from build123d import *

# Parameters (mm, degrees)
ESBO_O1_R                = 1.6
ESBO_O1_R_2              = 5.15
ESBO_O1_W                = 14.5
ESBO_O1_H                = 10
ESBO_O1_W_2              = 30.747802568
ESBO_O1_H_2              = 3
ESBO_O1_W_3              = 30.747802569
RESSALTO_EXTRUS_O1_DEPTH = 7
RESSALTO_EXTRUS_O3_START = 7
ESBO_O1_5_W              = 30.747802569
ESBO_O1_5_H              = 3
ESBO_O1_5_W_2            = 30.747802568
RESSALTO_EXTRUS_O3_DEPTH = 5


with BuildPart() as part:
    # Esboço1 → Ressalto-extrusão1 (new body)
    # profile 1 of 5: a face of its own
    with BuildSketch(Plane.XY):
        Polygon((60.087398189, 33.548797322), (-59.912601811, 33.548797322), (-59.912601811, 26.644004496), (-29.164799242, 26.644004496), (-29.164799242, 23.644004496), (-59.912601811, 23.644004496), (-59.912601811, -30.686339735), (-29.164799242, -30.686339735), (-29.164799242, -33.686339735), (-59.912601811, -33.686339735), (-59.912601811, -40.591132561), (60.087398189, -40.591132561), (60.087398189, -33.686339735), (29.339595621, -33.686339735), (29.339595621, -30.686339735), (60.087398189, -30.686339735), (60.087398189, 23.644004496), (29.339595621, 23.644004496), (29.339595621, 26.644004496), (60.087398189, 26.644004496), align=None)
        with Locations((-47.375288378, -37.09616762)):
            Circle(ESBO_O1_R, mode=Mode.SUBTRACT)
        with Locations((0.087398189, -37.13140726)):
            Circle(ESBO_O1_R, mode=Mode.SUBTRACT)
        with Locations((-39.912601811, -21.441132561)):
            Circle(ESBO_O1_R_2, mode=Mode.SUBTRACT)
        with Locations((47.550084756, -37.09616762)):
            Circle(ESBO_O1_R, mode=Mode.SUBTRACT)
        with Locations((40.087398189, -21.441132561)):
            Circle(ESBO_O1_R_2, mode=Mode.SUBTRACT)
        with Locations((-16.412601811, 3.558867439)):
            Circle(ESBO_O1_R_2, mode=Mode.SUBTRACT)
        with Locations((-47.375288378, 30.05383238)):
            Circle(ESBO_O1_R, mode=Mode.SUBTRACT)
        with Locations((-15.162601811, 21.548797322)):
            Rectangle(ESBO_O1_W, ESBO_O1_H, mode=Mode.SUBTRACT)
        with Locations((0.087398189, 30.08907202)):
            Circle(ESBO_O1_R, mode=Mode.SUBTRACT)
        with Locations((16.587398189, 3.558867439)):
            Circle(ESBO_O1_R_2, mode=Mode.SUBTRACT)
        with Locations((15.337398189, 21.548797322)):
            Rectangle(ESBO_O1_W, ESBO_O1_H, mode=Mode.SUBTRACT)
        with Locations((47.550084756, 30.05383238)):
            Circle(ESBO_O1_R, mode=Mode.SUBTRACT)
    # profile 2 of 5: a face of its own
    with BuildSketch(Plane.XY):
        Polygon((-29.164799242, -30.686339735), (-59.912601811, -30.686339735), (-59.912601811, -33.451202678), (-59.912601811, -33.686339735), (-29.164799242, -33.686339735), align=None)
    # profile 3 of 5: a face of its own
    with BuildSketch(Plane.XY):
        Polygon((60.087398189, -33.646676702), (60.087398189, -30.686339735), (29.339595621, -30.686339735), (29.339595621, -33.686339735), (60.087398189, -33.686339735), align=None)
    # profile 4 of 5: a face of its own
    with BuildSketch(Plane.XY):
        with Locations((44.713496905, 25.144004496)):
            Rectangle(ESBO_O1_W_2, ESBO_O1_H_2)
    # profile 5 of 5: a face of its own
    with BuildSketch(Plane.XY):
        with Locations((-44.538700527, 25.144004496)):
            Rectangle(ESBO_O1_W_3, ESBO_O1_H_2)
    extrude(amount=RESSALTO_EXTRUS_O1_DEPTH)

    # Esboço1<5> → Ressalto-extrusão3 (add)
    with BuildSketch(Plane.XY.offset(RESSALTO_EXTRUS_O3_START)):
        with Locations((-44.538700527, 25.144004496)):
            Rectangle(ESBO_O1_5_W, ESBO_O1_5_H)
        with Locations((44.713496905, 25.144004496)):
            Rectangle(ESBO_O1_5_W_2, ESBO_O1_5_H)
        Polygon((-29.164799242, -30.686339735), (-59.912601811, -30.686339735), (-59.912601811, -33.451202678), (-59.912601811, -33.686339735), (-29.164799242, -33.686339735), align=None)
        Polygon((60.087398189, -33.646676702), (60.087398189, -30.686339735), (29.339595621, -30.686339735), (29.339595621, -33.686339735), (60.087398189, -33.686339735), align=None)
    extrude(amount=RESSALTO_EXTRUS_O3_DEPTH)


solid = part.part
The listing builds one solid part. Answer for the finished solid, in the listing's coordinates (mm). A direction names the side the tool comes from. Give positions to 0.01 mm unless a question says otherwise; leave off trailing zeros. Write each loop counter-clockwise with the first axis right and the second up, starting at its lowest first coordinate (ties: lowest second). Pieces come first, ordered by that corner, then holes. Notation, with made-up numbers: (45.25, 32) -> (68.25, 32) arc R29 ccw to (68.25, 58) -> close; hole circle Ø6 at (39.25, -10). An arc over 180 degrees is marked (long way). One line per question, with ' | ' between items. Start each with the question number.
1. Section A-A (y = 20) is taken. Determine the outline of the cut face in (x, z).
2. Section C-C (x = -36.5) is taken. Determine the outline of the cut face in (y, z).
3. Given pin 1 Ø3 at (x, y) = (0.09, 30.09) entering from +Z; pin 2 Ø1.5 at (x, z) = (47.5, 10.5) entering from -Y; pin 3 Ø5 at (x, y) = (-47.38, 30.05) entering from +Z, each flat-ended and moving along its own axis, determine where each tip first touches the part or whether it passes through.
4. For faces 1 (the flat face through (15, 26.549, 3)), 2 (the flat face through (44, 25, 12)), 3 (the flat face through (-29.165, 25, 9)), 4 (the flat face through (44, -33.686, 9)), 5 (the flat face through (44, 26.644, 9)), determine the directions among +Z, -Z, +X, -X, +Y, -Y from which every point of the face is accessible in a straight line to the end or side of a thin tool.
5. Section D-D (x = 13) is taken. Determine the outline of the cut face in (y, z).
6. For a pull along X with two mould halves and no side action, classify faces 6 (the cylindrical face through (49.028, -37.709, 3.451)), 7 (the cylindrical face through (-0.121, 31.675, 3.451)), 8 (the flat face through (44, 23.644, 9)), 9 (the flat face through (-59.913, -4, 3)) as pulls with the +X half, pulls with the -X half, needs draft (parallel to the pull), parting line crosses it, or undercut.
7. Section B-B (z = 9) is taken. Determine the outline of the cut face in (x, y).
8. Find the intervals of material crossed by probe 1 along X at (y, z) = (25.5, 4.25); probe 2 along X at (y, z) = (2.5, 2.75); probe 3 along Y at (x, z) = (-1, 6.25), in increasing order.
Response values:
1) outline: (-59.91, 0) -> (-22.41, 0) -> (-22.41, 7) -> (-59.91, 7) -> close; (-7.91, 0) -> (8.09, 0) -> (8.09, 7) -> (-7.91, 7) -> close; (22.59, 0) -> (60.09, 0) -> (60.09, 7) -> (22.59, 7) -> close
2) outline: (-40.59, 0) -> (-25.3, 0) -> (-25.3, 7) -> (-30.69, 7) -> (-30.69, 12) -> (-33.69, 12) -> (-33.69, 7) -> (-40.59, 7) -> close; (-17.58, 0) -> (33.55, 0) -> (33.55, 7) -> (26.64, 7) -> (26.64, 12) -> (23.64, 12) -> (23.64, 7) -> (-17.58, 7) -> close
3) pin 1: through | pin 2: y = -33.69 | pin 3: z = 7
4) face 1: +Z, -Z | face 2: +Z, +X, -X, +Y, -Y | face 3: +Z, +Y, -Y | face 4: +Z, +X, -X, -Y | face 5: +Z, +X, -X, +Y
5) outline: (-40.59, 0) -> (-0.14, 0) -> (-0.14, 7) -> (-40.59, 7) -> close; (7.25, 0) -> (16.55, 0) -> (16.55, 7) -> (7.25, 7) -> close; (26.55, 0) -> (33.55, 0) -> (33.55, 7) -> (26.55, 7) -> close
6) face 6: undercut | face 7: undercut | face 8: needs draft | face 9: pulls with the -X half
7) outline: (-59.91, -33.69) -> (-29.16, -33.69) -> (-29.16, -30.69) -> (-59.91, -30.69) -> close; (-59.91, 23.64) -> (-29.16, 23.64) -> (-29.16, 26.64) -> (-59.91, 26.64) -> close; (29.34, -33.69) -> (60.09, -33.69) -> (60.09, -30.69) -> (29.34, -30.69) -> close; (29.34, 23.64) -> (60.09, 23.64) -> (60.09, 26.64) -> (29.34, 26.64) -> close
8) probe 1: -59.91 to -22.41, -7.91 to 8.09, 22.59 to 60.09 | probe 2: -59.91 to -21.45, -11.37 to 11.55, 21.63 to 60.09 | probe 3: -40.59 to -38.31, -35.96 to 28.92, 31.26 to 33.55
